from build123d import *

# Parameters (mm, degrees)
BOSS_EXTRUDE1_DEPTH = 5
SKETCH2_W           = 2.5
SKETCH2_H           = 9.100970889
BOSS_EXTRUDE2_DEPTH = 5
CUT_EXTRUDE1_REACH  = 56.95
SKETCH3_R           = 2.7
SKETCH4_W           = 20
SKETCH4_H           = 5
SKETCH4_R           = 2.7
BOSS_EXTRUDE3_DEPTH = 5
SKETCH5_R           = 5
CUT_EXTRUDE2_DEPTH  = 10


with BuildPart() as part:
    # Sketch1 → Boss-Extrude1 (new body)
    with BuildSketch(Plane(origin=(0, 0, 0), x_dir=(1, 0, 0), z_dir=(0, 1, 0))):
        with BuildLine():
            Line((0, -25), (0, -40))
            Line((0, -40), (2.5, -40))
            Line((2.5, -40), (2.5, -30.899029111))
            ThreePointArc((2.5, -30.899029111), (19.044247329, -24.460511926), (29.342801502, -10))
            Line((29.342801502, -10), (37.342801502, -10))
            Line((37.342801502, -10), (37.342801502, 10))
            Line((37.342801502, 10), (29.342801502, 10))
            ThreePointArc((29.342801502, 10), (19.044247329, 24.460511926), (2.5, 30.899029111))
            Line((2.5, 30.899029111), (2.5, 40))
            Line((2.5, 40), (0, 40))
            Line((0, 40), (0, 25))
            ThreePointArc((0, 25), (25, 0), (0, -25))
        make_face()
    extrude(amount=BOSS_EXTRUDE1_DEPTH)

    # Sketch2 → Boss-Extrude2 (add)
    with BuildSketch(Plane.XZ):
        with Locations((1.25, 35.449514556)):
            Rectangle(SKETCH2_W, SKETCH2_H)
        with Locations((1.25, -35.449514556)):
            Rectangle(SKETCH2_W, SKETCH2_H)
    extrude(amount=BOSS_EXTRUDE2_DEPTH)

    # Sketch3 → Cut-Extrude1 (cut, up to next)
    with BuildSketch(Plane.ZY, mode=Mode.PRIVATE) as cut_extrude1_sk1:
        with Locations((-35.449514555, 0)):
            Circle(SKETCH3_R)
    cut_extrude1_tool1 = extrude(cut_extrude1_sk1.sketch, amount=-CUT_EXTRUDE1_REACH, mode=Mode.PRIVATE) & part.part
    # Sketch3 → Cut-Extrude1 (cut, up to next)
    with BuildSketch(Plane.ZY, mode=Mode.PRIVATE) as cut_extrude1_sk2:
        with Locations((35.449514555, 0)):
            Circle(SKETCH3_R)
    cut_extrude1_tool2 = extrude(cut_extrude1_sk2.sketch, amount=-CUT_EXTRUDE1_REACH, mode=Mode.PRIVATE) & part.part
    add(cut_extrude1_tool1.solids().sort_by_distance((0, 0, -35.449515))[0], mode=Mode.SUBTRACT)
    add(cut_extrude1_tool2.solids().sort_by_distance((0, 0, 35.449515))[0], mode=Mode.SUBTRACT)

    # Sketch4 → Boss-Extrude3 (add)
    with BuildSketch(Plane(origin=(37.342801502, 0, 0), x_dir=(0, 0, -1), z_dir=(1, 0, 0))):
        with BuildLine():
            add(Edge.make_bspline(
                [(-23.175620272, 7), (-37.080992454, -9.500000022), (3e-08, -9.5)],
                knots=[2.757195879, 2.757195879, 2.757195879, 4.712388982, 4.712388982, 4.712388982], degree=2, weights=[1, 0.559016994, 1]))
            add(Edge.make_bspline(
                [(3e-08, -9.5), (25, -9.499999986), (25, 2.5)],
                knots=[4.712388982, 4.712388982, 4.712388982, 6.283185307, 6.283185307, 6.283185307], degree=2, weights=[1, 0.707106782, 1]))
            add(Edge.make_bspline(
                [(25, 2.5), (25, 4.835206052), (23.175620272, 7)],
                knots=[0, 0, 0, 0.384396774, 0.384396774, 0.384396774], degree=2, weights=[1, 0.981586677, 1]))
            Line((23.175620272, 7), (-23.175620272, 7))
        make_face()
        with Locations((0, 2.5)):
            Rectangle(SKETCH4_W, SKETCH4_H, mode=Mode.SUBTRACT)
        with Locations((-19.5, 2.5)):
            Circle(SKETCH4_R, mode=Mode.SUBTRACT)
        with Locations((19.5, 2.5)):
            Circle(SKETCH4_R, mode=Mode.SUBTRACT)
        with Locations((0, -4.5)):
            Circle(SKETCH4_R, mode=Mode.SUBTRACT)
    extrude(amount=-BOSS_EXTRUDE3_DEPTH)

    # Sketch5 → Cut-Extrude2 (cut)
    with BuildSketch(Plane.ZY.offset(-32.342801502)):
        with Locations((-20, -7.759289568)):
            Circle(SKETCH5_R)
        with Locations((20, -7.759289568)):
            Circle(SKETCH5_R)
    extrude(amount=-CUT_EXTRUDE2_DEPTH, mode=Mode.SUBTRACT)


solid = part.part
Read the model definition and answer for the solid it produces. Units are mm, in the model's axes. A direction names the side the tool comes from. Coordinates: 2 decimals unless noted, no trailing zeros. Loops run counter-clockwise (first coordinate to the right, second up) from the corner with the lowest first, then second, coordinate; pieces in that order, holes last.
Q1. The mould has two halves that part along X. Classify faces 1 (the face through (19.243, 2.465, -24.305)), 2 (the face through (1, 0, -40)), 3 (the face through (2.5, 2, -33)): +X half, -X half, draft (parallel to the pull), parting line (faces both ways), or undercut.
Q2. The part is cut by section C-C on x = 9. Write down the section's boundary in (y, z).
Q3. The part is cut by section D-D on x = 26. Write down the section's boundary in (y, z), and give its area (3 significant figures).
Q4. Which of the six approach directions +Z, -Z, +X, -X, +Y, -Y give full straight-line access (tool end or side, diameter ignored) to faces 4 (the face through (2.5, -2, 33)), 5 (the face through (31, 2, 10)), 6 (the face through (1, -2, -30.899)), 7 (the face through (34.878, 1.466, 17.006))?
Q5. The part is cut by section B-B on z = 19.5. Write down the section's boundary in (x, y).
Q6. Consider probe 1 along Y at (x, z) = (36, 0); probe 2 along X at (y, z) = (1.5, -33); probe 3 along Y at (x, z) = (27.5, -9.5). Determine where each line is inside the solid, lowest interval first.
Q7. The part is cut by section A-A on x = 13.5. Write down the section's boundary in (y, z), and give its area (3 significant figures).
Q8. Each of these flat-tipped pins is pushed along its axis until it touches: pin 1 Ø3.5 at (x, y) = (30.5, 2.5) entering from +Z; pin 2 Ø3 at (x, y) = (10, -0.5) entering from -Z; pin 3 Ø3 at (y, z) = (-2.5, -17.5) entering from -X. Where does it stop, or does it pass through?
Results below:
1. face 1: undercut
1. face 2: draft
1. face 3: +X half
2. outline: (0, -29.66) - (5, -29.66) - (5, -23.32) - (0, -23.32) - close; (0, 23.32) - (5, 23.32) - (5, 29.66) - (0, 29.66) - close
3. outline: (0, -16.88) - (5, -16.88) - (5, 16.88) - (0, 16.88) - close
3. area: 169 mm2
4. face 4: +Z, +X, +Y, -Y
4. face 5: +Z, +Y, -Y
4. face 6: +X, -X, -Y
4. face 7: +X
5. outline: (15.64, 0) - (24.1, 0) - (24.1, 5) - (15.64, 5) - close; (32.34, -2.78) - (37.34, -2.78) - (37.34, -0.2) - (32.34, -0.2) - close; (32.34, 5.2) - (37.34, 5.2) - (37.34, 7) - (32.34, 7) - close
6. probe 1: y = -9.5 to -7.2, -1.8 to 7
6. probe 2: x = 0 to 2.5
6. probe 3: y = 0 to 5
7. outline: (0, -27.91) - (5, -27.91) - (5, -21.04) - (0, -21.04) - close; (0, 21.04) - (5, 21.04) - (5, 27.91) - (0, 27.91) - close
7. area: 68.6 mm2
8. pin 1: stops at z = 11.59
8. pin 2: stops at z = -29.79
8. pin 3: stops at x = 32.34
